Here's how the part is built. I have some questions about the finished solid (model axes, mm). A direction names the side the tool comes from. Give positions to 0.01 mm unless a question says otherwise; leave off trailing zeros. Order: outer loops, then holes, each group sorted by start corner. A loop starts at its lowest first (then second) coordinate and runs counter-clockwise, first axis right, second up. Notation, with made-up numbers: M 1.5,8 L 23.5,8 A19 cw 23.5,41 Z; hole C -9.5,-29.75 d2. An arc over 180 degrees is marked long. Use CSV: the item, a comma, the result in double quotes. Start each with the question number.
Autodesk Inventor part; units mm, degrees
ref_plane "YZ Plane" through (0, 0, 0) normal (1, 0, 0) x (0, 1, 0)
ref_plane "XZ Plane" through (0, 0, 0) normal (0, 1, 0) x (-1, 0, 0)
ref_plane "XY Plane" through (0, 0, 0) normal (0, 0, 1) x (1, 0, 0)
sketch "Sketch1" plane through (0, 0, 0) normal (0, 0, 1) x (1, 0, 0)
  circle A0 centre (0, 15.825) radius 9.125
  line L0 (-12.375, 0) -> (12.375, 0)
  arc A1 (12.375, 15.825) -> (-12.375, 15.825) centre (0, 15.825) ccw
  line L1 (12.375, 0) -> (12.375, 15.825)
  line L2 (-12.375, 0) -> (-12.375, 15.825)
  point P0 (0, 0)
  point P1 (0, 0)
  point P2 (0, 0)
  point P3 (0, 3.45)
  dimension "d28" = 18.25
  dimension "d29" = 24.75
  dimension "d30" = 24.75
  dimension "d31" = 3.45
sketch "Sketch2" plane through (0, 0, 0) normal (0, 1, 0) x (-1, 0, 0)
  line L0 (12.375, 0) -> (-12.375, 0)
  line L1 (-12.375, 0) -> (-12.375, -50)
  line L2 (-12.375, -50) -> (12.375, -50)
  line L3 (12.375, -50) -> (12.375, 0)
  point P0 (0, 0)
  point P1 (-12.375, 0)
  dimension "d5" = 24.75
  dimension "d10" = 50
extrude "Extrusion4" add sketch "Sketch2" along normal blind 2
extrude "Extrusion5" add sketch "Sketch1" against normal blind 2
fillet "Fillet1" radius 0.5 2 edges at (0, 0, 0) (0, 2, -2)
properties part number "Dudukan Proximity V2"
Q1. Imagine slicing it at C-C, the plane z = -26. Please give me the cut outline in (x, y) (3 decimals), then the cut area to 3 significant figures.
Q2. For faces 1 (the face through (0, 2, -26)), 2 (the face through (0, 1, -50)), which set-ups out of +Z, -Z, +X, -X, +Y, -Y let a thin tool reach every point of the face, with its end or its side?
Q3. Imagine slicing it at D-D, the plane x = 3. Please give me the cut outline in (y, z), then the cut area to 3 significant figures.
Q4. We'd pull the mould along X, two halves only. Please class faces 3 (the face through (4.906, 23.519, -0.986)), 4 (the face through (3, 7, -2)), 5 (the face through (0.272, 28.197, -0.986)), 6 (the face through (12.375, 1, -19)): pulls with the +X half, pulls with the -X half, needs draft (parallel to the pull), parting line crosses it, or undercut.
Q5. For P1, Ø8, axis at x = 2.5, z = -11.5, coming from the +Y side; P2, Ø12, axis at y = 12, z = -24, coming from the +X side; P3, Ø5, axis at x = 1, y = 5.5, coming from the -Z side, each with a flat end and sliding along its axis, tell me the tip position at first contact or that it passes through.
Q6. Imagine slicing it at B-B, the plane y = 9.75. Please give me the cut outline in (x, z) (3 decimals).
Q7. Imagine slicing it at A-A, the plane x = 0. Please give me the cut outline in (y, z), then the cut area to 3 significant figures.
Q8. I need wall thicknesses on line 1 (Y direction, x = 0, z = -0.9); line 2 (Y direction, x = -5.25, z = -46.5); line 3 (Z direction, x = 7.25, y = 4.25). Which ranges of each line are inside material? Lowest first, please. Write a range as [from, to].
Reply:
1,outline,"M -12.375,0 L 12.375,0 L 12.375,2 L -12.375,2 Z"
1,area,"49.5 mm^2"
2,face 1,"-Z, +X, -X, +Y"
2,face 2,"-Z, +X, -X, +Y, -Y"
3,outline,"M 0,-50 L 2,-50 L 2,-2.5 A0.5 cw 2.5,-2 L 7.21,-2 L 7.21,0 L 0.5,0 A0.5 ccw 0,-0.5 Z; M 24.44,-2 L 27.83,-2 L 27.83,0 L 24.44,0 Z"
3,area,"117 mm^2"
4,face 3,"undercut"
4,face 4,"needs draft"
4,face 5,"parting line crosses it"
4,face 6,"pulls with the +X half"
5,P1,"stops at y = 2"
5,P2,"passes through"
5,P3,"stops at z = -2"
6,outline,"M -12.375,-2 L -6.809,-2 L -6.809,0 L -12.375,0 Z; M 6.809,-2 L 12.375,-2 L 12.375,0 L 6.809,0 Z"
7,outline,"M 0,-50 L 2,-50 L 2,-2.5 A0.5 cw 2.5,-2 L 6.7,-2 L 6.7,0 L 0.5,0 A0.5 ccw 0,-0.5 Z; M 24.95,-2 L 28.2,-2 L 28.2,0 L 24.95,0 Z"
7,area,"116 mm^2"
8,line 1,"y = [0, 6.7], [24.95, 28.2]"
8,line 2,"y = [0, 2]"
8,line 3,"z = [-2, 0]"
